Solid Edge part; units mm, degrees
sketch "Sketch1" plane through (0, 0, 0) normal (0, 0, 1) x (1, 0, 0)
  line L0 (-82.5, -68.43) -> (82.5, -68.43)
  line L1 (82.5, -68.43) -> (82.5, 68.43)
  line L2 (82.5, 68.43) -> (-82.5, 68.43)
  line L3 (-82.5, 68.43) -> (-82.5, -68.43)
  dimension "D1" = 82.5
  dimension "D2" = 82.5
extrude "Extrusionsausprägung_1" add sketch "Sketch1" along normal blind 3
sketch "Sketch2" plane through (0, 0, 3) normal (0, 0, 1) x (1, 0, 0)
  line L0 (-82.5, -68.43) -> (-42.5, -68.43)
  line L1 (-42.5, -68.43) -> (-42.5, -33.43)
  line L2 (-42.5, -33.43) -> (-82.5, -33.43)
  line L3 (-82.5, -33.43) -> (-82.5, -68.43)
  dimension "D1" = 42.5
  dimension "D2" = 42.5
extrude "Cutout1" cut sketch "Sketch2" against normal through all
sketch "Sketch3" plane through (0, 0, 0) normal (0, 0, -1) x (-1, 0, 0)
  line L0 (-82.5, 68.43) -> (82.5, 68.43)
  line L1 (82.5, 68.43) -> (82.5, 38.43)
  line L2 (82.5, 38.43) -> (-82.5, 38.43)
  line L3 (-82.5, 38.43) -> (-82.5, 68.43)
  dimension "D1" = 82.5
  dimension "D2" = 82.5
extrude "Extrusionsausprägung_2" add sketch "Sketch3" along normal blind 3
sketch "Sketch4" plane through (-82.5, 17.5, 0) normal (-1, 0, 0) x (0, 1, 0)
  line L0 (50.93, 0) -> (30.93, 0)
  line L1 (30.93, 0) -> (30.93, -3)
  line L2 (30.93, -3) -> (50.93, -3)
  line L3 (50.93, -3) -> (50.93, 0)
  dimension "D1" = 30.93
  dimension "D2" = 50.93
extrude "Cutout2" cut sketch "Sketch4" against normal through all
sketch "Sketch5" plane through (0, -15, 0) normal (0, 0, -1) x (1, 0, 0)
  line L0 (-42.5, 53.43) -> (82.5, 53.43)
  line L1 (82.5, 53.43) -> (82.5, 34.9466)
  line L2 (82.5, 34.9466) -> (-42.5, 34.9466)
  line L3 (-42.5, 34.9466) -> (-42.5, 53.43)
extrude "Extrusionsausprägung_3" add sketch "Sketch5" along normal blind 6
sketch "Sketch6" plane through (0, 0, 3) normal (0, 0, 1) x (1, 0, 0)
  circle A0 centre (42.5, 58.43) radius 2.25
  circle A1 centre (42.5, -58.43) radius 2.25
  circle A2 centre (-12.5, -58.43) radius 2.25
  circle A3 centre (-42.5, 58.43) radius 2.25
  dimension "D1" = 42.5
  dimension "D2" = 42.5
  dimension "D3" = 42.5
extrude "Extrusionsausschnitt_1" cut sketch "Sketch6" against normal blind 245.2559
chamfer "Fase_1" distance 0.5 angle 60 4 edges at (-14.75, -58.43, 3) (40.25, -58.43, 3) (42.5, 56.18, 0) (-42.5, 56.18, 0) measured on face at (-56.65, -8.8314, 3)
properties material "Nylon, allgemein"
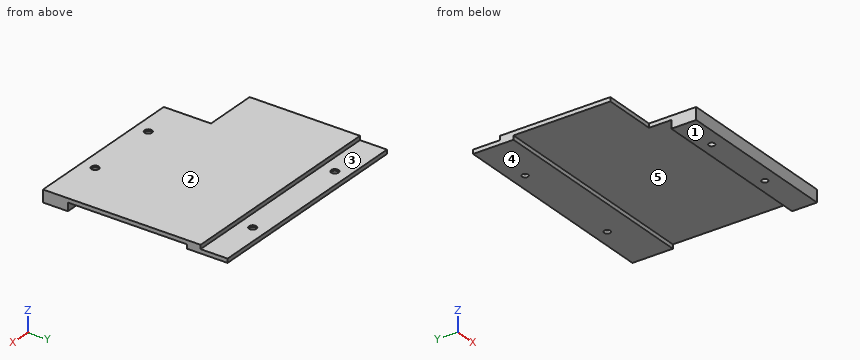
Geometry check sheet. Reference: the model listing, model coordinates, mm. Face numbers are marked on the shaded views. A direction names the side the tool comes from. Give positions to 0.01 mm unless a question says otherwise; leave off trailing zeros. Write each loop counter-clockwise with the first axis right and the second up, starting at its lowest first coordinate (ties: lowest second). Pieces come first, ordered by that corner, then holes.
1) Access from +Z, -Z, +X, -X, +Y, -Y to the whole of each face (thin tool, end or side, straight path). Record for the marked faces 1, 2, 3, 4 and 5.
2) Gauge pin test, flat ends, axial feed: pin 1 (1 mm diameter, centred on x = 22.5, y = 52.5, fed in from +Z); pin 2 (2.5 mm diameter, centred on y = -44.5, z = -0.5, fed in from -X); pin 3 (12 mm diameter, centred on x = 4.5, y = 32, fed in from -Z); pin 4 (2.5 mm diameter, centred on x = -12.5, y = -58.43, fed in from -Z) (3 decimals). Record the tip position at first contact, or that the pin passes through.
3) Section check A-A, the plane x = -12.5. Record the boundary of the cut face in (y, z), and give its area (3 significant figures).
4) Material ranges on L1, parallel to Y at x = 42.5, z = -2.25; L2, parallel to Y at x = -12.5, z = -0.5; L3, parallel to Y at x = -5, z = -1, recorded low to high.
5) Section check B-B, the plane y = 58.43. Record the boundary of the cut face in (x, z).
6) Section check D-D, the plane y = -58.43. Record the boundary of the cut face in (x, z).
7) Section check C-C, the plane x = 42.5. Record the boundary of the cut face in (y, z), and give its area (3 significant figures).
Computed:
1. face 1: -Z, +X, -X, +Y, -Y
1. face 2: +Z, +X, -X, +Y, -Y
1. face 3: +Z, +X, -X, +Y
1. face 4: -Z, +X, -X, +Y
1. face 5: -Z, +X, -X
2. pin 1: stops at z = 0
2. pin 2: stops at x = -42.5
2. pin 3: stops at z = 0
2. pin 4: passes through
3. outline: (-68.43, -6) - (-60.68, -6) - (-60.68, 2.13) - (-61.18, 3) - (-68.43, 3) - close; (-56.18, -6) - (-49.95, -6) - (-49.95, 0) - (38.43, 0) - (38.43, -3) - (68.43, -3) - (68.43, 0) - (48.43, 0) - (48.43, 3) - (-55.68, 3) - (-56.18, 2.13) - close
3. area: 511 mm2
4. L1: y = -68.43 to -60.68, -56.18 to -49.95, 38.43 to 56.18, 60.68 to 68.43
4. L2: y = -68.43 to -60.68, -56.18 to -49.95, 38.43 to 68.43
4. L3: y = -68.43 to -49.95, 38.43 to 68.43
5. outline: (-82.5, -3) - (-44.75, -3) - (-44.75, -0.87) - (-45.25, 0) - (-82.5, 0) - close; (-40.25, -3) - (40.25, -3) - (40.25, -0.87) - (39.75, 0) - (-39.75, 0) - (-40.25, -0.87) - close; (44.75, -3) - (82.5, -3) - (82.5, 0) - (45.25, 0) - (44.75, -0.87) - close
6. outline: (-42.5, -6) - (-14.75, -6) - (-14.75, 2.13) - (-15.25, 3) - (-42.5, 3) - close; (-10.25, -6) - (40.25, -6) - (40.25, 2.13) - (39.75, 3) - (-9.75, 3) - (-10.25, 2.13) - close; (44.75, -6) - (82.5, -6) - (82.5, 3) - (45.25, 3) - (44.75, 2.13) - close
7. outline: (-68.43, -6) - (-60.68, -6) - (-60.68, 2.13) - (-61.18, 3) - (-68.43, 3) - close; (-56.18, -6) - (-49.95, -6) - (-49.95, 0) - (38.43, 0) - (38.43, -3) - (56.18, -3) - (56.18, -0.87) - (55.68, 0) - (48.43, 0) - (48.43, 3) - (-55.68, 3) - (-56.18, 2.13) - close; (60.68, -3) - (68.43, -3) - (68.43, 0) - (61.18, 0) - (60.68, -0.87) - close
7. area: 497 mm2
